Build history of the part. All positions in model axes, mm. Face numbers are marked on the shaded views. A direction names the side the tool comes from. Coordinates: 2 decimals unless noted, no trailing zeros. Order: outer loops, then holes, each group sorted by start corner. A loop starts at its lowest first (then second) coordinate and runs counter-clockwise, first axis right, second up. Notation, with made-up numbers: (18.5, -0.75) - (27.5, -0.75) arc R23 cw to (27.5, 16.25) - close; hole circle Ø10 at (-28, 83.5). An arc over 180 degrees is marked (long way). One line per item, written item: value.
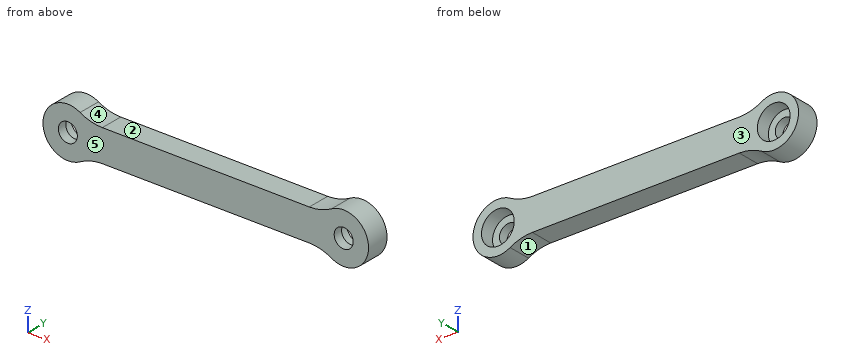
from build123d import *

# Parameters (mm, degrees)
SKETCH1_R           = 2.1
BOSS_EXTRUDE1_DEPTH = 5
SKETCH2_R           = 3.625
CUT_EXTRUDE1_DEPTH  = 3
FILLET1_R           = 10


with BuildPart() as part:
    # Sketch1 → Boss-Extrude1 (new body)
    with BuildSketch(Plane(origin=(0, 0, 0), x_dir=(1, 0, 0), z_dir=(0, 1, 0))):
        with BuildLine():
            Line((-56.757359313, -3.5), (-4.242640687, -3.5))
            ThreePointArc((-4.242640687, -3.5), (5.5, 0), (-4.242640687, 3.5))
            Line((-4.242640687, 3.5), (-56.757359313, 3.5))
            ThreePointArc((-56.757359313, 3.5), (-66.5, 0), (-56.757359313, -3.5))
        make_face()
        with Locations(Location((-61, 0, 0), (0, 0, 270))):
            Circle(SKETCH1_R, mode=Mode.SUBTRACT)
        with Locations(Location((0, 0, 0), (0, 0, 90))):
            Circle(SKETCH1_R, mode=Mode.SUBTRACT)
    extrude(amount=BOSS_EXTRUDE1_DEPTH)

    # Sketch2 → Cut-Extrude1 (cut)
    with BuildSketch(Plane(origin=(0, 5, 0), x_dir=(1, 0, 0), z_dir=(0, 1, 0))):
        with Locations(Location((-61, 0, 0), (0, 0, 270))):
            Circle(SKETCH2_R)
        with Locations(Location((0, 0, 0), (0, 0, 270))):
            Circle(SKETCH2_R)
    extrude(amount=-CUT_EXTRUDE1_DEPTH, mode=Mode.SUBTRACT)

    # Fillet1
    fillet1_edges = [part.edges().sort_by_distance(p)[0] for p in [
        (-4.242640687, 2.5, 3.5),
        (-56.757359313, 2.5, 3.5),
        (-56.757359313, 2.5, -3.5),
        (-4.242640687, 2.5, -3.5),
    ]]
    fillet(fillet1_edges, radius=FILLET1_R)


solid = part.part
1. 3-axis set-ups, long thin cutter, end or side, ignore diameter. For the marked faces 1, 2 and 3: which of +Z, -Z, +X, -X, +Y, -Y reach the whole face in a straight line?
Values found:
face 1: -Z, +Y, -Y
face 2: +Z, +Y, -Y
face 3: +Z, -Z, +X, -X, +Y
2. Probe line 1 along X through (y, z) = (1, 0); line 2 along X through (y, z) = (3.9, 0) (3 decimals); line 3 along Z through (x, y) = (-61, 0.5). List the from-to ranges inside material, lowest first.
Values found:
line 1: x = -66.5 to -63.1, -58.9 to -2.1, 2.1 to 5.5
line 2: x = -66.5 to -64.625, -57.375 to -3.625, 3.625 to 5.5
line 3: z = -5.5 to -2.1, 2.1 to 5.5
3. Band-saw the part on A-A, the plane y = 3.95. Give the cut face in (x, z) (3 decimals).
Values found:
outline: (-58.298, -4.79) arc R10 cw to (-53.384, -3.5) - (-7.616, -3.5) arc R10 cw to (-2.702, -4.79) arc R5.5 ccw (long way) to (-2.702, 4.79) arc R10 cw to (-7.616, 3.5) - (-53.384, 3.5) arc R10 cw to (-58.298, 4.79) arc R5.5 ccw (long way) to start; hole circle Ø7.25 at (-61, 0); hole circle Ø7.25 at (0, 0)
4. Band-saw the part on D-D, the plane y = 0.8. Give the cut face in (x, z).
Values found:
outline: (-58.3, -4.79) arc R10 cw to (-53.38, -3.5) - (-7.62, -3.5) arc R10 cw to (-2.7, -4.79) arc R5.5 ccw (long way) to (-2.7, 4.79) arc R10 cw to (-7.62, 3.5) - (-53.38, 3.5) arc R10 cw to (-58.3, 4.79) arc R5.5 ccw (long way) to start; hole circle Ø4.2 at (-61, 0); hole circle Ø4.2 at (0, 0)
5. Band-saw the part on B-B, the plane x = -61. Give the cut face in (y, z) (3 decimals), and give its area (4 significant figures).
Values found:
outline: (0, -5.5) - (5, -5.5) - (5, -3.625) - (2, -3.625) - (2, -2.1) - (0, -2.1) - close; (0, 2.1) - (2, 2.1) - (2, 3.625) - (5, 3.625) - (5, 5.5) - (0, 5.5) - close
area: 24.85 mm2
6. Flat gauge pins, fed straight in: P1, Ø2, axis at y = 2.5, z = -2, coming from the -X side; P2, Ø3, axis at y = 4, z = 2, coming from the +X side; P3, Ø2, axis at x = -21, y = 1.5, coming from the +Z side; P4, Ø2.5, axis at x = 0, z = 0, coming from the -Y side. Where does each tip first touch, or does it go through?
Values found:
P1: stops at x = -66.41
P2: stops at x = 5.48
P3: stops at z = 3.5
P4: passes through
7. Two-plate mould, pull along X, no slides. Class the marked faces 4 and 5: pulls with the +X half, pulls with the -X half, needs draft (parallel to the pull), parting line crosses it, or undercut.
Values found:
face 4: undercut
face 5: needs draft
8. Band-saw the part on C-C, the plane z = 1.5. Give the cut face in (x, y), and give its area (3 significant figures).
Values found:
outline: (-66.29, 0) - (-62.47, 0) - (-62.47, 2) - (-64.3, 2) - (-64.3, 5) - (-66.29, 5) - close; (-59.53, 0) - (-1.47, 0) - (-1.47, 2) - (-3.3, 2) - (-3.3, 5) - (-57.7, 5) - (-57.7, 2) - (-59.53, 2) - close; (1.47, 0) - (5.29, 0) - (5.29, 5) - (3.3, 5) - (3.3, 2) - (1.47, 2) - close
area: 307 mm2
